Verification items for the finished model (mm, model axes). A direction names the side the tool comes from. Round coordinates to 2 decimals unless told otherwise and drop trailing zeros. Write each loop counter-clockwise with the first axis right and the second up, starting at its lowest first coordinate (ties: lowest second). Pieces come first, ordered by that corner, then holes. Notation, with made-up numbers: M 64,84 L 84,84 A33 cw 84,117 Z; hole C 63.25,-10 d4. An arc over 180 degrees is marked long. One line per item, written item: value. Start each with the question number.
Item 1: Gauge pin test, flat end, axial feed: pin 1 (1 mm diameter, centred on x = -11.5, z = -5, fed in from +Y). Record the tip position at first contact, or that the pin passes through.
Item 2: Section check A-A, the plane z = 1.75. Record the cut outline in (x, y).
Item 3: Section check C-C, the plane x = -2. Record the cut outline in (y, z), then the cut area to 3 significant figures.
Item 4: Draft check along Y on faces 4 (the face through (0, 6, -7.5)), 5 (the face through (15, 3.75, 0)), 6 (the face through (0, 0, 0)). Enter one of: +Y half, -Y half, draft (parallel to the pull), parting line (faces both ways), or undercut.
Item 5: Thickness scan on probe 1 along Z at (x, y) = (-4, 8.75); probe 2 along X at (y, z) = (6.25, 5.25); probe 3 along Y at (x, z) = (14, 0.25). Record the ranges inside material, lowest first. Write a range as from..to.
Item 6: Tool access check on faces 1 (the face through (-15, 5.25, 0)), 2 (the face through (-14.5, 6, 0)), 3 (the face through (16, 6, 0)). Record the directions out of +Z, -Z, +X, -X, +Y, -Y that give a thin tool (end or side, any length) a straight path to the whole face; none if there is none.
Item 7: Section check D-D, the plane y = 9.25. Record the cut outline in (x, z).
Item 8: Section check B-B, the plane y = 4.75. Record the cut outline in (x, z), then the cut area to 4 significant figures.
from build123d import *

# Parameters (mm, degrees)
SKETCH1_W           = 32
SKETCH1_H           = 18
BOSS_EXTRUDE1_DEPTH = 10
SHELL1_T            = -1.5
SKETCH3_W           = 5.5
SKETCH3_H           = 1.5
CUT_EXTRUDE1_DEPTH  = 35.713109915


with BuildPart() as part:
    # Sketch1 → Boss-Extrude1 (new body)
    with BuildSketch(Plane(origin=(0, 0, 0), x_dir=(1, 0, 0), z_dir=(0, 1, 0))):
        Rectangle(SKETCH1_W, SKETCH1_H)
    extrude(amount=BOSS_EXTRUDE1_DEPTH)

    # Shell1
    shell1_openings = [part.faces().sort_by_distance(p)[0] for p in [
        (0, 10, 0),
    ]]
    offset(amount=SHELL1_T, openings=shell1_openings, kind=Kind.INTERSECTION)

    # Sketch3 → Cut-Extrude1 (cut, through all)
    with BuildSketch(Plane(origin=(16, 0, 0), x_dir=(0, 0, -1), z_dir=(1, 0, 0))):
        with Locations((0, 4.5)):
            Rectangle(SKETCH3_W, SKETCH3_H)
    extrude(amount=-CUT_EXTRUDE1_DEPTH, mode=Mode.SUBTRACT)


solid = part.part
Response values:
1. pin 1: stops at y = 1.5
2. outline: M -16,0 L 16,0 L 16,3.75 L 14.5,3.75 L 14.5,1.5 L -14.5,1.5 L -14.5,3.75 L -16,3.75 Z; M -16,5.25 L -14.5,5.25 L -14.5,10 L -16,10 Z; M 14.5,5.25 L 16,5.25 L 16,10 L 14.5,10 Z
3. outline: M 0,-9 L 10,-9 L 10,-7.5 L 1.5,-7.5 L 1.5,7.5 L 10,7.5 L 10,9 L 0,9 Z
3. area: 52.5 mm2
4. face 4: draft
4. face 5: undercut
4. face 6: -Y half
5. probe 1: z = -9..-7.5, 7.5..9
5. probe 2: x = -16..-14.5, 14.5..16
5. probe 3: y = 0..1.5
6. face 1: +X, -X
6. face 2: +Y
6. face 3: +Z, -Z, +X, +Y, -Y
7. outline: M -16,-9 L 16,-9 L 16,9 L -16,9 Z; hole M -14.5,-7.5 L 14.5,-7.5 L 14.5,7.5 L -14.5,7.5 Z
8. outline: M -16,-9 L 16,-9 L 16,-2.75 L 14.5,-2.75 L 14.5,-7.5 L -14.5,-7.5 L -14.5,-2.75 L -16,-2.75 Z; M -16,2.75 L -14.5,2.75 L -14.5,7.5 L 14.5,7.5 L 14.5,2.75 L 16,2.75 L 16,9 L -16,9 Z
8. area: 124.5 mm2
